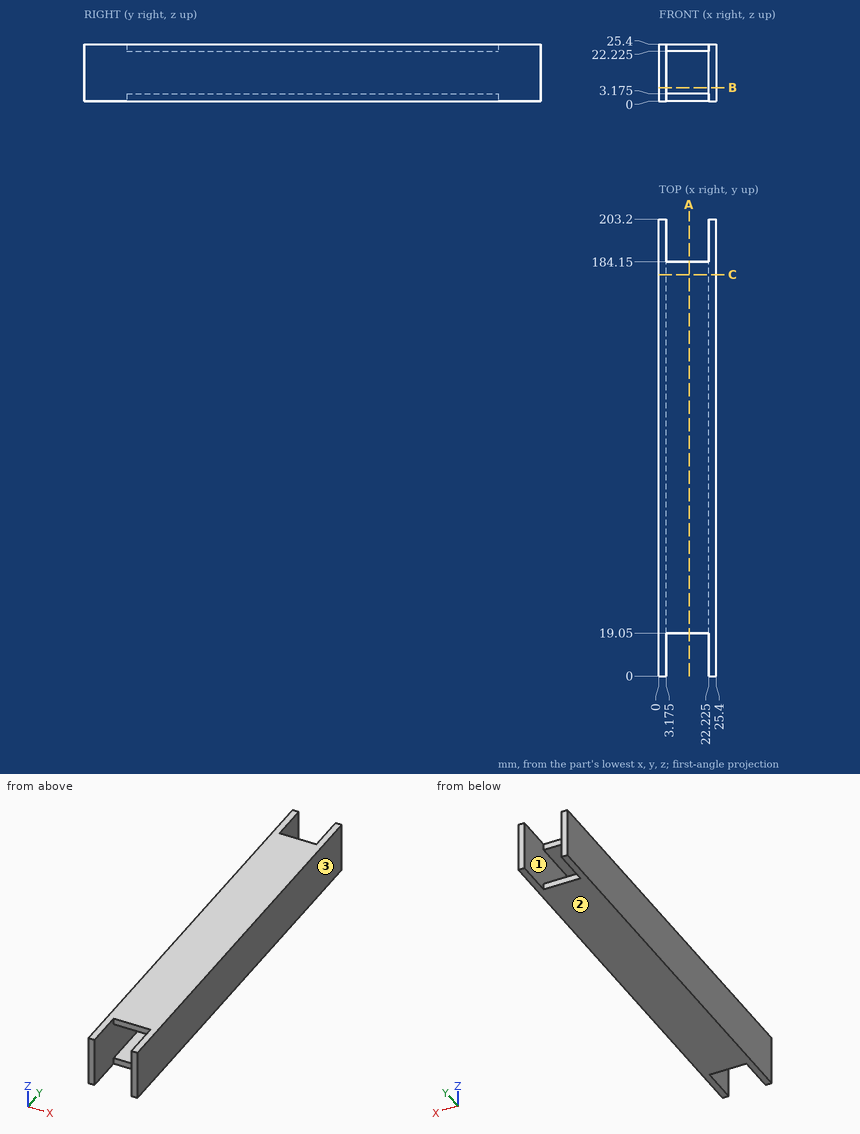
Here's the drawing with two shaded views (mm, measured from the low corner). I have some questions. Give positions to 0.01 mm unless a question says otherwise; leave off trailing zeros. Loops run counter-clockwise (first coordinate to the right, second up) from the corner with the lowest first, then second, coordinate; pieces in that order, holes last. Notation, with made-up numbers: (75, -37) - (111, -37) arc R28 cw to (111, -10) - close; hole circle Ø7 at (-17, 57). An arc over 180 degrees is marked (long way). Answer in a Markdown table with one row per item. Add a question column.
Q1. If we section it at A-A (x = 13.5): List the corners of the cut face in (y, z) for me (3 decimals), plus the area to 3 significant figures.
Q2. If we section it at C-C (y = 178.5): List the corners of the cut face in (x, z) for me (3 decimals).
Q3. If we section it at B-B (z = 6): List the corners of the cut face in (x, y) for me (3 decimals), plus the area to 3 significant figures.
Q4. Please list where these lines run through material, in increasing order: L1, parallel to Z at x = 19, y = 42.5 (3 decimals); L2, parallel to Y at x = 14.5, z = 22.5. Write a range as from..to.
Q5. We'd pull the mould along X, two halves only. Please class the marked faces 1, 2 and 3: +X half, -X half, draft (parallel to the pull), parting line (faces both ways), or undercut.
Q6. For pin 1 (8 mm diameter, centred on x = 18, z = 5, fed in from -Y); pin 2 (3 mm diameter, centred on y = 87.5, z = 9, fed in from -X); pin 3 (1 mm diameter, centred on x = 16, z = 1, fed in from +Y), each with a flat end and sliding along its axis, tell me the tip position at first contact or that it passes through.
The answers:
| question | item | result |
|---|---|---|
| 1 | outline | (19.05, 0) - (184.15, 0) - (184.15, 3.175) - (19.05, 3.175) - close; (19.05, 22.225) - (184.15, 22.225) - (184.15, 25.4) - (19.05, 25.4) - close |
| 1 | area | 1,050 mm^2 |
| 2 | outline | (0, 0) - (25.4, 0) - (25.4, 25.4) - (0, 25.4) - close; hole (3.175, 3.175) - (22.225, 3.175) - (22.225, 22.225) - (3.175, 22.225) - close |
| 3 | outline | (0, 0) - (3.175, 0) - (3.175, 203.2) - (0, 203.2) - close; (22.225, 0) - (25.4, 0) - (25.4, 203.2) - (22.225, 203.2) - close |
| 3 | area | 1,290 mm^2 |
| 4 | L1 | z = 0..3.175, 22.225..25.4 |
| 4 | L2 | y = 19.05..184.15 |
| 5 | face 1 | undercut |
| 5 | face 2 | draft |
| 5 | face 3 | +X half |
| 6 | pin 1 | stops at y = 19.05 |
| 6 | pin 2 | stops at x = 0 |
| 6 | pin 3 | stops at y = 184.15 |
